```python
from build123d import *

# Parameters (mm, degrees)
SKETCH_2_W      = 3
SKETCH_2_H      = 6
EXTRUDE_1_DEPTH = 3


with BuildPart() as part:
    # 草图2 → 凸台-拉伸1 (new body)
    with BuildSketch(Plane.XY):
        with BuildLine():
            Line((2.047890023, 48.855305477), (8, 48.855305477))
            Line((8, 48.855305477), (8, 51.855305477))
            Line((8, 51.855305477), (16, 51.855305477))
            Line((16, 51.855305477), (16, 8.855305477))
            Line((16, 8.855305477), (8, 8.855305477))
            Line((8, 8.855305477), (8, 5.855305477))
            Line((8, 5.855305477), (0.390512484, 5.855305477))
            ThreePointArc((0.390512484, 5.855305477), (0, 8.905305477), (-0.390512484, 5.855305477))
            Line((-0.390512484, 5.855305477), (-8, 5.855305477))
            Line((-8, 5.855305477), (-8, 8.855305477))
            Line((-8, 8.855305477), (-16, 8.855305477))
            Line((-16, 8.855305477), (-16, 51.855305477))
            Line((-16, 51.855305477), (-8, 51.855305477))
            Line((-8, 51.855305477), (-8, 48.855305477))
            Line((-8, 48.855305477), (-2.047890023, 48.855305477))
            Line((-2.047890023, 48.855305477), (-2.047890023, 43.855305477))
            Line((-2.047890023, 43.855305477), (-4, 43.855305477))
            Line((-4, 43.855305477), (-4, 40.855305477))
            Line((-4, 40.855305477), (-2, 40.855305477))
            Line((-2, 40.855305477), (-2, 36.855305477))
            Line((-2, 36.855305477), (2, 36.855305477))
            Line((2, 36.855305477), (2, 40.855305477))
            Line((2, 40.855305477), (4, 40.855305477))
            Line((4, 40.855305477), (4, 43.855305477))
            Line((4, 43.855305477), (2.047890023, 43.855305477))
            Line((2.047890023, 43.855305477), (2.047890023, 48.855305477))
        make_face()
        with Locations((-11.5, 23.355305477)):
            Rectangle(SKETCH_2_W, SKETCH_2_H, mode=Mode.SUBTRACT)
    extrude(amount=EXTRUDE_1_DEPTH)


solid = part.part
```
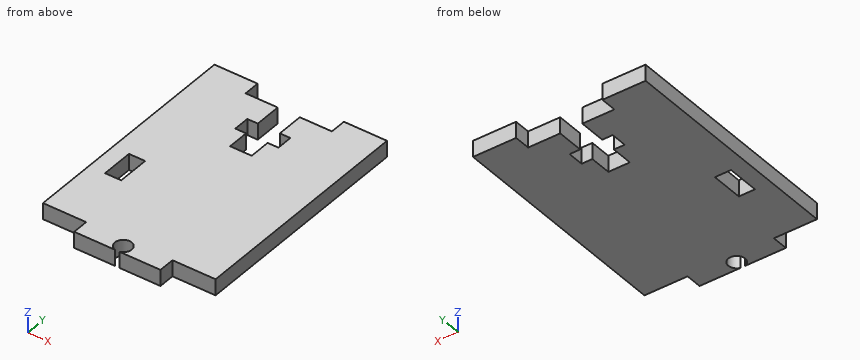
Check sheet for the modelled part. Datum: model origin and axes. Units: mm. Round coordinates to 2 decimals unless told otherwise and drop trailing zeros. Write each loop counter-clockwise with the first axis right and the second up, starting at its lowest first coordinate (ties: lowest second). Pieces come first, ordered by that corner, then holes. Notation, with made-up numbers: M 7,25 L 65,25 A22 ccw 65,46 Z; hole C 86.25,82.25 d4. An arc over 180 degrees is marked long. Write item = value, one per line. Start each with the question number.
1. Scan lines: line 1 (X direction, y = 43, z = 1); line 2 (X direction, y = 47, z = 1.6); line 3 (Y direction, x = -11, z = 0.2). Record each from-to range of solid material in increasing order. Write a range as [from, to].
2. Gauge pin test, flat ends, axial feed: pin 1 (3 mm diameter, centred on x = 0, y = 7.36, fed in from +Z); pin 2 (1.5 mm diameter, centred on x = 10, z = 1.5, fed in from -Y); pin 3 (0.6 mm diameter, centred on x = 3, z = 1, fed in from +Y). Record the tip position at first contact, or that the pin passes through.
3. Section check A-A, the plane x = -11. Record the cut outline in (y, z).
4. Section check C-C, the plane x = -3. Record the cut outline in (y, z).
Results found:
q1.line_1 = [-16, -4], [4, 16]
q1.line_2 = [-16, -2.05], [2.05, 16]
q1.line_3 = [8.86, 20.36], [26.36, 51.86]
q2.pin_1 = through
q2.pin_2 = 8.86
q2.pin_3 = 48.86
q3.outline = M 8.86,0 L 20.36,0 L 20.36,3 L 8.86,3 Z; M 26.36,0 L 51.86,0 L 51.86,3 L 26.36,3 Z
q4.outline = M 5.86,0 L 40.86,0 L 40.86,3 L 5.86,3 Z; M 43.86,0 L 48.86,0 L 48.86,3 L 43.86,3 Z
